Build history of the part. All positions in model axes, mm. Give positions to 0.01 mm unless a question says otherwise; leave off trailing zeros. Order: outer loops, then holes, each group sorted by start corner. A loop starts at its lowest first (then second) coordinate and runs counter-clockwise, first axis right, second up. Notation, with made-up numbers: (31.5, 85.5) - (61.5, 85.5) arc R25 cw to (61.5, 99.5) - close; hole circle Ø8 at (16.25, 85.25). An arc over 180 degrees is marked (long way). Answer in a Markdown table with one row per item.
```python
from build123d import *

# Parameters (mm, degrees)
SKETCH1_W           = 8.5
SKETCH1_H           = 8.5
BOSS_EXTRUDE1_DEPTH = 3.2
CUT_EXTRUDE1_DEPTH  = 3.05
CUT_EXTRUDE2_DEPTH  = 0.15


with BuildPart() as part:
    # Sketch1 → Boss-Extrude1 (new body)
    with BuildSketch(Plane(origin=(0, 0, 0), x_dir=(1, 0, 0), z_dir=(0, 1, 0))):
        with Locations((4.25, -4.25)):
            Rectangle(SKETCH1_W, SKETCH1_H)
    extrude(amount=BOSS_EXTRUDE1_DEPTH)

    # Sketch2 → Cut-Extrude1 (cut)
    with BuildSketch(Plane(origin=(0, 3.2, 0), x_dir=(1, 0, 0), z_dir=(0, 1, 0))):
        Polygon((1.5, -8.5), (0, -7), (0, -8.5), align=None)
        Polygon((0, -1.5), (1.5, 0), (0, 0), align=None)
        Polygon((8.5, 0), (7, 0), (8.5, -1.5), align=None)
        Polygon((8.5, -8.5), (8.5, -7), (7, -8.5), align=None)
    extrude(amount=-CUT_EXTRUDE1_DEPTH, mode=Mode.SUBTRACT)

    # Sketch3 → Cut-Extrude2 (cut)
    with BuildSketch(Plane.XZ):
        Polygon((8.5, 1.13137085), (7.969669914, 1.661700936), (6.838299064, 0.530330086), (7.36862915, 0), (1.13137085, 0), (1.661700936, 0.530330086), (0.530330086, 1.661700936), (0, 1.13137085), (0, 7.36862915), (0.530330086, 6.838299064), (1.661700936, 7.969669914), (1.13137085, 8.5), (7.36862915, 8.5), (6.838299064, 7.969669914), (7.969669914, 6.838299064), (8.5, 7.36862915), align=None)
    extrude(amount=-CUT_EXTRUDE2_DEPTH, mode=Mode.SUBTRACT)


solid = part.part
```
1. Cut at B-B on z = 2.75. Write the cut outline in (x, y), and give its area (3 significant figures).
Check result:
| item | result |
|---|---|
| outline | (0, 0.15) - (8.5, 0.15) - (8.5, 3.2) - (0, 3.2) - close |
| area | 25.9 mm² |
2. Probe line 1 (Y direction, x = 3.75, z = 5); line 2 (Z direction, x = 7.5, y = 0.65); line 3 (X direction, y = 2.95, z = 0.75). List the from-to ranges inside material, lowest first.
Check result:
| item | result |
|---|---|
| line 1 | y = 0.15 to 3.2 |
| line 2 | z = 0.5 to 8 |
| line 3 | x = 0.75 to 7.75 |
3. Two-plate mould, pull along X, no slides. Class faces 1 (the face through (1, 2, 8)), 2 (the face through (4, 0.15, 4)), 3 (the face through (8, 0, 8)), 4 (the face through (8.5, 2, 4)): +X half, -X half, draft (parallel to the pull), parting line (faces both ways), or undercut.
Check result:
| item | result |
|---|---|
| face 1 | -X half |
| face 2 | undercut |
| face 3 | draft |
| face 4 | +X half |
4. Cut at C-C on x = 5. Write the cut outline in (y, z).
Check result:
| item | result |
|---|---|
| outline | (0.15, 0) - (3.2, 0) - (3.2, 8.5) - (0.15, 8.5) - close |
5. Cut at A-A on y = 2.1. Write the cut outline in (x, z).
Check result:
| item | result |
|---|---|
| outline | (0, 1.5) - (1.5, 0) - (7, 0) - (8.5, 1.5) - (8.5, 7) - (7, 8.5) - (1.5, 8.5) - (0, 7) - close |
6. Drop flat-ended pins along their axis: P1, Ø1.4, axis at x = 0.5, z = 8, coming from the +Y side; P2, Ø2.5, axis at x = 6, z = 6, coming from the -Y side. Give the stop position or say it passes through.
Check result:
| item | result |
|---|---|
| P1 | stops at y = 3.2 |
| P2 | stops at y = 0.15 |
